For this review, take the finished solid that the model builds, in its own axes (mm). A direction names the side the tool comes from. Coordinates: 2 decimals unless noted, no trailing zeros. Loops run counter-clockwise (first coordinate to the right, second up) from the corner with the lowest first, then second, coordinate; pieces in that order, holes last.
1. Mouldability with a two-part tool opening along Y and no side actions: class faces 6 (the face through (-13, -11, 0)), 7 (the face through (-13, -5.379, -4)), 8 (the face through (-13.03, -6.62, -6.44)) as pulls with the +Y half, pulls with the -Y half, needs draft (parallel to the pull), parting line crosses it, or undercut.
2. Take a section at D-D, the plane y = -7.75. State the section outline as (x, z) points, then the cut area to 3 significant figures.
3. Machinability: for faces 1 (the face through (-10.879, -6.6, -3.5)), 2 (the face through (-13, -4, 0)), 3 (the face through (-15.121, -8.4, -3.5)), 4 (the face through (-13, -9.621, -4)), 5 (the face through (-13.03, -8.38, -6.44)), which of the approach directions +Z, -Z, +X, -X, +Y, -Y give a long, thin tool a straight path to every point of the face, cutting with its end or side? Answer none if there is none.
4. Take a section at A-A, the plane z = -8.5. State the section outline as (x, y) points, then the cut area to 3 significant figures.
5. Clearance check with flat-ended pins moving along their axes: P1, Ø1.5, axis at x = -12.5, z = -4, coming from the +Y side; P2, Ø0.8, axis at x = -12, z = -10.5, coming from the -Y side; P3, Ø1.5, axis at x = -12, y = -5, coming from the +Z side. State where each tip first meets the part, or that it passes through.
6. Take a section at B-B, the plane x = -12.65. State the section outline as (y, z) points, then the cut area to 3 significant figures.
7. Take a section at C-C, the plane y = -10. State the section outline as (x, z) points, then the cut area to 3 significant figures.
8. To check wall thickness, follow probe 1 along Y at (x, z) = (-14.2, -0.5); probe 2 along Y at (x, z) = (-14.45, -8.25); probe 3 along Y at (x, z) = (-11.85, -7.5). State the ranges of each line that lie inside material, in increasing order.
Autodesk Inventor part; units mm, degrees
ref_plane "YZ Plane" through (0, 0, 0) normal (1, 0, 0) x (0, 1, 0)
ref_plane "XZ Plane" through (0, 0, 0) normal (0, 1, 0) x (-1, 0, 0)
ref_plane "XY Plane" through (0, 0, 0) normal (0, 0, 1) x (1, 0, 0)
ref_plane "Work Plane1" through (0, 0, 0) normal (0, 0, 1) x (1, 0, 0)
sketch "Sketch1" plane through (0, 0, 0) normal (0, 0, 1) x (1, 0, 0)
  circle A0 centre (-13, -7.5) radius 3
  line L0 (-13, -7.5) -> (-10.8787, -9.6213) construction
  line L1 (-13, -7.5) -> (-10, -7.5) construction
  line L2 (-15.1213, -5.3787) -> (-10.8787, -5.3787)
  line L3 (-10.8787, -5.3787) -> (-10.8787, -9.6213)
  line L4 (-10.8787, -9.6213) -> (-15.1213, -9.6213)
  line L5 (-15.1213, -9.6213) -> (-15.1213, -5.3787)
  line L6 (-15.1213, -5.3787) -> (-10.8787, -9.6213) construction
  line L7 (-10.8787, -5.3787) -> (-15.1213, -9.6213) construction
  point P0 (0, 0)
  dimension "d0" = 45
extrude "Extrusion1" add sketch "Sketch1" against normal blind 12 contours L3 L4 L5 L2
sketch "Sketch2" plane through (0, 0, 0) normal (0, 0, 1) x (1, 0, 0)
  circle A0 centre (-13, -7.5) radius 3
  line L0 (-10.8787, -11.5) -> (-15.1213, -11.5)
  line L1 (-15.1213, -11.5) -> (-15.1213, -3.5)
  line L2 (-15.1213, -3.5) -> (-10.8787, -3.5)
  line L3 (-10.8787, -3.5) -> (-10.8787, -11.5)
  line L4 (-10.8787, -11.5) -> (-15.1213, -3.5) construction
  line L5 (-15.1213, -11.5) -> (-10.8787, -3.5) construction
  point P0 (0, 0)
  dimension "d3" = 8
extrude "Extrusion2" add sketch "Sketch2" along normal blind 2 contours L3 A0 L1 | A0 L1 L2 L3 | L3 L0 L1 A0
fillet "Fillet1" radius 4 2 edges at (-13, -3.5, 2) (-13, -11.5, 2)
sketch "Sketch3" plane through (-15.1213, -9.6213, -12) normal (-1, 0, 0) x (0, 0, 1)
  line L0 (4, 9.5928) -> (4, -5.4072)
  line L1 (12, 0) -> (0, 0)
  arc A0 (0, 0) -> (4, 0) centre (2, 2.2361) ccw
  line L2 (12, 4.2426) -> (0, 4.2426)
  arc A1 (4, 4.2426) -> (0, 4.2426) centre (2, 2.0066) ccw
  point P0 (12, 9.6213)
  dimension "d7" = 3
  dimension "d8" = 3
extrude "Extrusion3" add sketch "Sketch3" against normal up to surface (4.2426 mm away)
sketch "Sketch4" plane through (-15.1213, -5.3787, 0) normal (-1, 0, 0) x (0, 0, 1)
  line L0 (-14, -3.3713) -> (-10, -3.3713)
  line L1 (-10, -3.3713) -> (-10, -0.8713)
  line L2 (-10, -0.8713) -> (-14, -0.8713)
  line L3 (-14, -0.8713) -> (-14, -3.3713)
  line L4 (-12, -4.2426) -> (-12, 0)
  line L5 (-14, -3.3713) -> (-10, -0.8713) construction
  line L6 (-10, -3.3713) -> (-14, -0.8713) construction
  line L7 (-10, -3.3713) -> (-2.7742, -2.6186)
  line L8 (2, -1.5854) -> (2, -2.6572)
  line L9 (-10, -0.8713) -> (-2.7742, -1.624)
  arc A0 (-2.7742, -2.6186) -> (-2.7742, -1.624) centre (-2.826, -2.1213) ccw
  point P0 (0, 5.3787)
  point P1 (-12, -2.1213)
  point P2 (2, -2.1213)
  dimension "d11" = 4
  dimension "d12" = 2.5
  dimension "d13" = 0.5
extrude "Extrusion4" cut sketch "Sketch4" against normal up to next
fillet "Fillet2" radius 0.5 2 edges at (-13, -6.25, -12) (-13, -8.75, -12)
properties part number "fastener"
Results list:
1. face 6: needs draft
1. face 7: pulls with the +Y half
1. face 8: undercut
2. outline: (-15.12, -2.39) - (-10.88, -2.39) - (-10.88, 2) - (-15.12, 2) - close
2. area: 18.6 mm2
3. face 1: +Z, -Z, +X, +Y, -Y
3. face 2: +X, -X, +Y
3. face 3: +Z, -Z, -X, +Y, -Y
3. face 4: +X, -X, -Y
3. face 5: -Z, +X, -X
4. outline: (-15.12, -9.98) - (-10.88, -9.98) - (-10.88, -8.59) - (-15.12, -8.59) - close; (-15.12, -6.41) - (-10.88, -6.41) - (-10.88, -5.02) - (-15.12, -5.02) - close
4. area: 11.8 mm2
5. P1: stops at y = -5.38
5. P2: stops at y = -10.38
5. P3: stops at z = 1.81
6. outline: (-11.5, 0) - (-9.62, 0) - (-9.62, -8) arc R3 ccw to (-9.62, -12) - (-9.25, -12) arc R0.5 ccw to (-8.75, -11.5) - (-8.75, -10) - (-8, -2.77) arc R0.5 cw to (-7, -2.77) - (-6.25, -10) - (-6.25, -11.5) arc R0.5 ccw to (-5.75, -12) - (-5.38, -12) arc R3 ccw to (-5.38, -8) - (-5.38, 0) - (-3.5, 0) arc R4 ccw to (-6.96, 2) - (-8.04, 2) arc R4 ccw to start
6. area: 49.0 mm2
7. outline: (-15.12, -11.47) - (-10.88, -11.47) - (-10.88, -8.53) - (-15.12, -8.53) - close; (-15.12, 0) - (-10.88, 0) - (-10.88, 1.48) - (-15.12, 1.48) - close
7. area: 18.8 mm2
8. probe 1: y = -9.62 to -5.38
8. probe 2: y = -9.82 to -8.57, -6.43 to -5.18
8. probe 3: y = -9.62 to -8.49, -6.51 to -5.38
